Here's how the part is built. I have some questions about the finished solid (model axes, mm). A direction names the side the tool comes from. Coordinates: 2 decimals unless noted, no trailing zeros. Write each loop counter-clockwise with the first axis right and the second up, starting at its lowest first coordinate (ties: lowest second). Pieces come first, ordered by that corner, then holes. Notation, with made-up numbers: M -31,36.25 L 1,36.25 A22 cw 1,65.25 Z; hole C -8,52.5 d5. An arc over 180 degrees is marked long. Use one line per item in the form item = value. Start each with the question number.
1. Please list where these lines run through material, in increasing order: line 1 along Y through (x, z) = (-42.05, 8); line 2 along Y through (x, z) = (-7.5, -8); line 3 along Z through (x, y) = (-4.5, 8). Write a range as [from, to].
2. I want a section at A-A, the plane y = 8. List the corners of the cut face in (x, z) for me, plus the area to 3 significant figures.
3. I want a section at D-D, the plane x = -22. List the corners of the cut face in (y, z) for me.
4. I want a section at B-B, the plane x = -4.5. List the corners of the cut face in (y, z) for me (1 decimal).
5. I want a section at C-C, the plane z = -8. List the corners of the cut face in (x, y) for me.
6. On a 3-axis mill with a long thin cutter (end or side, diameter ignored), from which of +Z, -Z, +X, -X, +Y, -Y can I reach the whole of each face in a straight line? I mean faces 1 (the face through (0, 11.4, -8.1)), 2 (the face through (-44.97, 10.22, -4.85)), 3 (the face through (-39, 8, 4)), 4 (the face through (-1.75, 2, -8)). Say none if no direction works.
7. Thinking about a two-plate mould opening in Z: for faces 5 (the face through (-21.2, 0.57, -15.4)), 6 (the face through (-0.9, 14, -10.4)), 7 (the face through (-47, 8, -6)), which applies, released by +Z, released by -Z, zero draft, split by the parting line, or undercut?
8. I'm going to push flat-ended pins straight in: pin 1 Ø5 at (y, z) = (9, -8.5) entering from +X; pin 2 Ø8 at (y, z) = (8, 8) entering from +X; pin 3 Ø1 at (x, y) = (-28, 12.5) entering from +Z; pin 4 Ø1.4 at (y, z) = (14, -7.5) entering from +X. Where does each tip first touch, or does it pass through?
Autodesk Inventor part; units mm, degrees
ref_plane "Work Plane1" through (-39, 0, 16) normal (-1, 0, 0) x (0, 0, 1)
ref_plane "YZ Plane" through (0, 0, 0) normal (1, 0, 0) x (0, 1, 0)
ref_plane "XZ Plane" through (0, 0, 0) normal (0, 1, 0) x (-1, 0, 0)
sketch "Sketch1" plane through (0, 0, 0) normal (0, 1, 0) x (-1, 0, 0)
  line L0 (43, 16) -> (43, -16)
  line L1 (43, -16) -> (0, -16)
  line L2 (0, -16) -> (0, 0)
  line L3 (0, 0) -> (23, 0)
  line L4 (39, 16) -> (39, 16)
  line L5 (39, 16) -> (43, 16)
  arc A0 (23, 0) -> (39, 16) centre (23, 16) ccw
  dimension "d0" = 16
  dimension "d1" = 32
  dimension "d2" = 4
  dimension "d3" = 16
  dimension "d4" = 43
extrude "Extrusion1" add sketch "Sketch1" along normal blind 16
fillet "Fillet1" radius 2 6 edges at (-34.3137, 16, 4.6863) (-11.5, 16, 0) (-21.5, 16, -16) (-21.5, 0, -16) (-34.3137, 0, 4.6863) (-11.5, 0, 0)
ref_plane "Work Plane1" through (-39, 0, 16) normal (-1, 0, 0) x (0, 0, 1)
sketch "Sketch2" plane through (-39, 0, 16) normal (-1, 0, 0) x (0, 0, 1)
  line L0 (-16, 14) -> (0, 14)
  line L1 (0, 2) -> (-16, 2)
  line L2 (-14, 14) -> (0, 14)
  line L3 (0, 14) -> (0, 2)
  line L4 (0, 2) -> (-14, 2)
  line L5 (-16, 4) -> (-16, 12)
  arc A0 (-14, 14) -> (-16, 12) centre (-14, 12) ccw
  arc A1 (-16, 4) -> (-14, 2) centre (-14, 4) ccw
  point P0 (-16, 0)
  dimension "d9" = 2
  dimension "d10" = 16
extrude "Extrusion2" cut sketch "Sketch2" against normal blind 16
sketch "Sketch3" plane through (-39, 0, 16) normal (1, 0, 0) x (0, 0, -1)
  line L0 (0, 0) -> (18, 0)
  line L1 (18, 16) -> (0, 16)
  line L2 (0, 2) -> (0, 14)
  point P0 (16, 0)
  point P1 (8, 8)
  dimension "d13" = 16
  dimension "d14" = 8
  dimension "d15" = 8
hole "Hole1" at (-39, 8, 8) direction (-1, 0, 0) diameter 6.756 depth 8.8
sketch "Sketch4" plane through (0, 0, -2) normal (1, 0, 0) x (0, 0, -1)
  line L0 (0, 16) -> (12, 16)
  line L1 (14, 2) -> (14, 14)
  line L2 (4.5, 14) -> (7.5, 14) construction
  line L3 (4.5, 13.1) -> (7.5, 13.1)
  line L4 (7.5, 14.9) -> (4.5, 14.9)
  arc A0 (4.5, 14.9) -> (4.5, 13.1) centre (4.5, 14) ccw
  arc A1 (7.5, 13.1) -> (7.5, 14.9) centre (7.5, 14) ccw
  line L5 (7.5, 2) -> (4.5, 2) construction
  line L6 (7.5, 2.9) -> (4.5, 2.9)
  line L7 (4.5, 1.1) -> (7.5, 1.1)
  arc A2 (7.5, 1.1) -> (7.5, 2.9) centre (7.5, 2) ccw
  arc A3 (4.5, 2.9) -> (4.5, 1.1) centre (4.5, 2) ccw
  point P0 (-2, 0)
  point P1 (6, 8)
  point P2 (6, 8)
  point P3 (6, 8)
  point P4 (6, 14)
  point P5 (6, 2)
  dimension "d23" = 8
  dimension "d24" = 8
  dimension "d62" = 0
  dimension "d63" = 1.8
  dimension "d64" = 12
  dimension "d65" = 6
  dimension "d66" = 1.8
  dimension "d67" = 3
  dimension "d68" = 0
  dimension "d69" = 3
extrude "Extrusion3" cut sketch "Sketch4" against normal blind 1.75
hole "Hole2" at (0, 8, -8) direction (-1, 0, 0) diameter 6.125 depth 19.05
sketch "Sketch5" plane through (-43, 0, 16) normal (-1, 0, 0) x (0, 0, 1)
  circle A0 centre (-22, 8) radius 2.5
  line L0 (-8, 8) -> (-22, 8) construction
  circle A1 centre (-8, 8) radius 3.378 construction
  point P0 (-16, 0)
  dimension "d42" = 14
  dimension "d43" = 5
extrude "Extrusion4" add sketch "Sketch5" along normal blind 4
equation "\"d1\" = 2 * d0"
equation "\"d66\" = d63"
equation "\"d69\" = d67"
properties part number "vive_mount"
Answer list:
q1.line_1 = [0, 4.62], [11.38, 16]
q1.line_2 = [0, 4.94], [11.06, 16]
q1.line_3 = [-16, -11.06], [-4.94, 0]
q2.outline = M -47,-8.5 L -43,-8.5 L -43,-16 L 0,-16 L 0,-11.06 L -19.05,-11.06 L -19.05,-4.94 L 0,-4.94 L 0,0 L -39,0 L -39,4.62 L -43,4.62 L -43,-3.5 L -47,-3.5 Z; M -43,11.38 L -39,11.38 L -39,16 L -43,16 Z
q2.area = 628 mm²
q3.outline = M 0,-14 A2 ccw 2,-16 L 14,-16 A2 ccw 16,-14 L 16,-2 A2 ccw 14,0 L 2,0 A2 ccw 0,-2 Z
q4.outline = M 0,-14 A2 ccw 2,-16 L 14,-16 A2 ccw 16,-14 L 16,-2 A2 ccw 14,0 L 2,0 A2 ccw 0,-2 Z; hole C 8,-8 d6.1
q5.outline = M -47,6.5 L -43,6.5 L -43,0 L 0,0 L 0,1.1 L -1.75,1.1 L -1.75,2.9 L 0,2.9 L 0,4.94 L -19.05,4.94 L -19.05,11.06 L 0,11.06 L 0,13.1 L -1.75,13.1 L -1.75,14.9 L 0,14.9 L 0,16 L -43,16 L -43,9.5 L -47,9.5 Z
q6.face_1 = +Z, -Z, +X, +Y, -Y
q6.face_2 = -X
q6.face_3 = +Z, +X
q6.face_4 = +X
q7.face_5 = released by -Z
q7.face_6 = undercut
q7.face_7 = zero draft
q8.pin_1 = 0
q8.pin_2 = -39
q8.pin_3 = 0.27
q8.pin_4 = -1.75
